Model file for the job. Use its own axes, mm. Face numbers are marked on the shaded views. Coordinates: 2 decimals unless noted, no trailing zeros. Write each loop counter-clockwise with the first axis right and the second up, starting at its lowest first coordinate (ties: lowest second). Pieces come first, ordered by that corner, then holes. Notation, with made-up numbers: (-27.5, -27) -> (-23.5, -27) arc R17 cw to (-23.5, -13) -> close; hole circle Ø11 at (49, -27). An arc over 180 degrees is marked (long way). Write item = value, one per line. Start each with the question number.
from build123d import *

# Parameters (mm, degrees)
SKETCH1_R               = 45
SKETCH1_R_2             = 2.25
SKETCH1_R_3             = 1.75
BOSS_EXTRUDE1_DEPTH     = 2.5
SKETCH2_R               = 29.85
SKETCH2_R_2             = 12.65
BOSS_EXTRUDE2_DEPTH     = 1
CUT_EXTRUDE1_DEPTH      = 64.688696014
CUT_EXTRUDE1_DEPTH_BACK = 64.688696014
SKETCH3_R               = 45
SKETCH3_R_2             = 12.5
FILLET1_R               = 0.5


with BuildPart() as part:
    # Sketch1 → Boss-Extrude1 (new body)
    with BuildSketch(Plane.XY):
        Circle(SKETCH1_R)
        Circle(SKETCH1_R_2, mode=Mode.SUBTRACT)
        with Locations((0, 33.5)):
            Circle(SKETCH1_R_3, mode=Mode.SUBTRACT)
        with Locations((33.5, 0)):
            Circle(SKETCH1_R_3, mode=Mode.SUBTRACT)
        with Locations((0, -33.5)):
            Circle(SKETCH1_R_3, mode=Mode.SUBTRACT)
        with Locations((-33.5, 0)):
            Circle(SKETCH1_R_3, mode=Mode.SUBTRACT)
    extrude(amount=BOSS_EXTRUDE1_DEPTH)

    # Sketch2 → Boss-Extrude2 (add)
    with BuildSketch(Plane(origin=(0, 0, 0), x_dir=(-1, 0, 0), z_dir=(0, 0, -1))):
        Circle(SKETCH2_R)
        Circle(SKETCH2_R_2, mode=Mode.SUBTRACT)
    extrude(amount=BOSS_EXTRUDE2_DEPTH)

    # Sketch3 → Cut-Extrude1 (cut, two sides: drawn at the far end of the back side and taken through both)
    with BuildSketch(Plane.XY.offset(-CUT_EXTRUDE1_DEPTH_BACK)):
        Circle(SKETCH3_R)
        Circle(SKETCH3_R_2, mode=Mode.SUBTRACT)
    extrude(amount=CUT_EXTRUDE1_DEPTH + CUT_EXTRUDE1_DEPTH_BACK, mode=Mode.SUBTRACT)

    # Fillet1
    fillet1_edges = [part.edges().sort_by_distance(p)[0] for p in [
        (-12.5, 0, 2.5),
        (-12.5, 0, 0),
        (-2.25, 0, 0),
        (-2.25, 0, 2.5),
    ]]
    fillet(fillet1_edges, radius=FILLET1_R)


solid = part.part
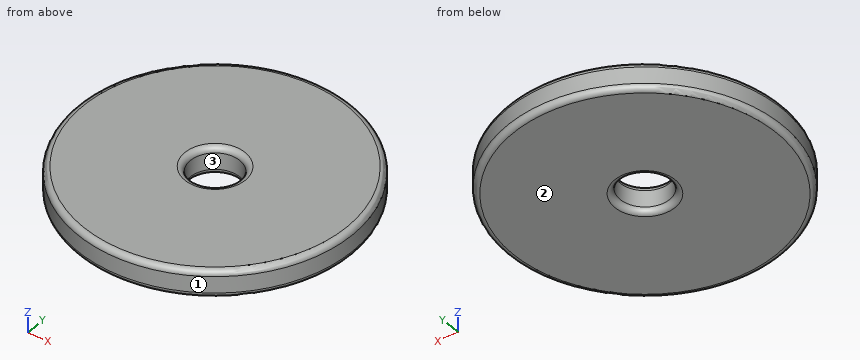
(1) Drill centre lines: line 1 along Y through (x, z) = (0, 1.05); line 2 along Y through (x, z) = (3.5, 1.3); line 3 along X through (y, z) = (0.5, 1.9). Where is each one in solid material? Low to high.
(2) Mould opens along Y. For the marked faces 1, 2 and 3 say: released by +Y, released by -Y, zero draft, split by the parting line, or undercut.
(3) Drop flat-ended pins along their axis: pin 1 Ø1 at (x, z) = (6.5, 2) entering from -Y; pin 2 Ø1.5 at (x, y) = (1.5, 7) entering from -Z. Give the stop position or say it passes through.
(4) Saw through at C-C (z = 1.2). Give the cut face in (x, y), then the cut area to 3 significant figures.
(5) Saw through at A-A (y = 0). Give the cut face in (x, z), then the cut area to 3 significant figures.
Returned:
q1.line_1 = -12.5 to -2.25, 2.25 to 12.5
q1.line_2 = -12 to 12
q1.line_3 = -12.49 to -2.19, 2.19 to 12.49
q2.face_1 = split by the parting line
q2.face_2 = zero draft
q2.face_3 = undercut
q3.pin_1 = -10.97
q3.pin_2 = 0
q4.outline = circle Ø25 at (0, 0); hole circle Ø4.5 at (0, 0)
q4.area = 475 mm2
q5.outline = (-12.5, 0.5) arc R0.5 ccw to (-12, 0) -> (-2.75, 0) arc R0.5 ccw to (-2.25, 0.5) -> (-2.25, 2) arc R0.5 ccw to (-2.75, 2.5) -> (-12, 2.5) arc R0.5 ccw to (-12.5, 2) -> close; (2.25, 0.5) arc R0.5 ccw to (2.75, 0) -> (12, 0) arc R0.5 ccw to (12.5, 0.5) -> (12.5, 2) arc R0.5 ccw to (12, 2.5) -> (2.75, 2.5) arc R0.5 ccw to (2.25, 2) -> close
q5.area = 50.8 mm2
